Study the drawing (mm; zero at the part's minimum x, y, z) and answer. A direction names the side the tool comes from. Round coordinates to 2 decimals unless told otherwise and drop trailing zeros. Write each loop counter-clockwise with the first axis right and the second up, starting at its lowest first coordinate (ties: lowest second). Pieces come first, ordered by that corner, then holes. Notation, with made-up numbers: (39, 70) - (55, 70) arc R26 cw to (55, 90) - close; hole circle Ø8 at (70, 80.5). An arc over 180 degrees is marked (long way). Return JSON: item names as keys, results as strings. Group by question number.
(1) Which of the six approach directions +Z, -Z, +X, -X, +Y, -Y give full straight-line access (tool end or side, diameter ignored) to the marked faces 1, 2 and 3?
(2) Section C-C, the plane y = 3 is taken. Write down the section's boundary in (x, z), then the cut area to 3 significant figures.
(3) Section A-A, the plane x = 22.5 is taken. Write down the section's boundary in (y, z), then the cut area to 3 significant figures.
(4) Find the intervals of material crossed by line 1 along Y through (x, z) = (37.5, 3.1); line 2 along Y through (x, z) = (22.5, 5.5); line 3 along Z through (x, y) = (31.5, 15), in increasing order. Write a range as [from, to].
(5) Section B-B, the plane y = 28 is taken. Write down the section's boundary in (x, z), then the cut area to 3 significant figures.
(6) Section D-D, the plane x = 10.5 is taken. Write down the section's boundary in (y, z), then the cut area to 3 significant figures.
(7) Each of these flat-tipped pins is pushed along its axis until it touches: pin 1 (4 mm diameter, centred on x = 22.5, y = 12, fed in from +Z); pin 2 (6.5 mm diameter, centred on x = 36, y = 28.5, fed in from +Z); pin 3 (4 mm diameter, centred on y = 11.5, z = 6, fed in from -X). Where does it stop, or does it pass through?
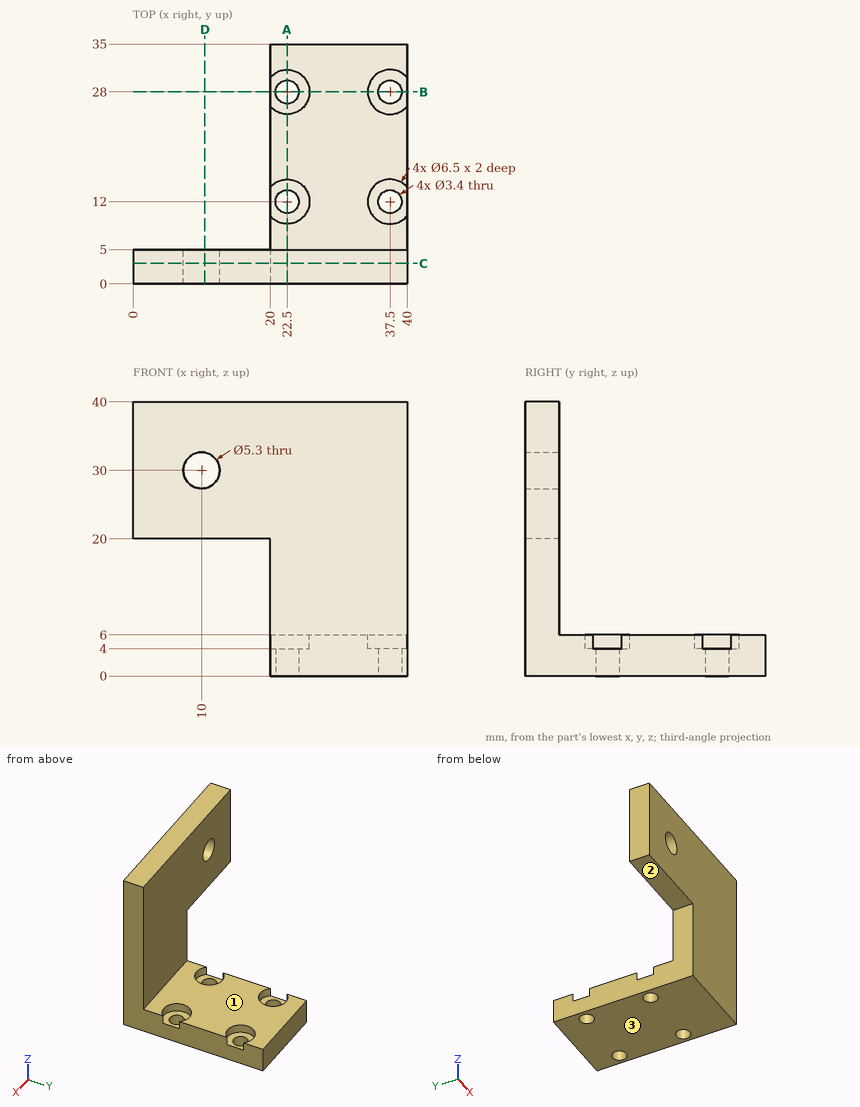
Working result:
{
 "1": {"face 1": "+Z, +X, -X, +Y", "face 2": "-Z, -X, +Y, -Y", "face 3": "-Z, +X, -X, +Y, -Y"},
 "2": {"outline": "(0, 20) - (20, 20) - (20, 0) - (40, 0) - (40, 40) - (0, 40) - close; hole circle Ø5.3 at (10, 30)", "area": "1,180 mm^2"},
 "3": {"outline": "(0, 0) - (10.3, 0) - (10.3, 4) - (8.75, 4) - (8.75, 6) - (5, 6) - (5, 40) - (0, 40) - close; (13.7, 0) - (26.3, 0) - (26.3, 4) - (24.75, 4) - (24.75, 6) - (15.25, 6) - (15.25, 4) - (13.7, 4) - close; (29.7, 0) - (35, 0) - (35, 6) - (31.25, 6) - (31.25, 4) - (29.7, 4) - close", "area": "327 mm^2"},
 "4": {"line 1": "y = [0, 10.3], [13.7, 26.3], [29.7, 35]", "line 2": "y = [0, 8.75], [15.25, 24.75], [31.25, 35]", "line 3": "z = [0, 6]"},
 "5": {"outline": "(20, 0) - (20.8, 0) - (20.8, 4) - (20, 4) - close; (24.2, 0) - (35.8, 0) - (35.8, 4) - (34.25, 4) - (34.25, 6) - (25.75, 6) - (25.75, 4) - (24.2, 4) - close; (39.2, 0) - (40, 0) - (40, 4) - (39.2, 4) - close", "area": "69.8 mm^2"},
 "6": {"outline": "(0, 20) - (5, 20) - (5, 27.4) - (0, 27.4) - close; (0, 32.6) - (5, 32.6) - (5, 40) - (0, 40) - close", "area": "74.0 mm^2"},
 "7": {"pin 1": "stops at z = 4", "pin 2": "stops at z = 6", "pin 3": "stops at x = 20"}
}
